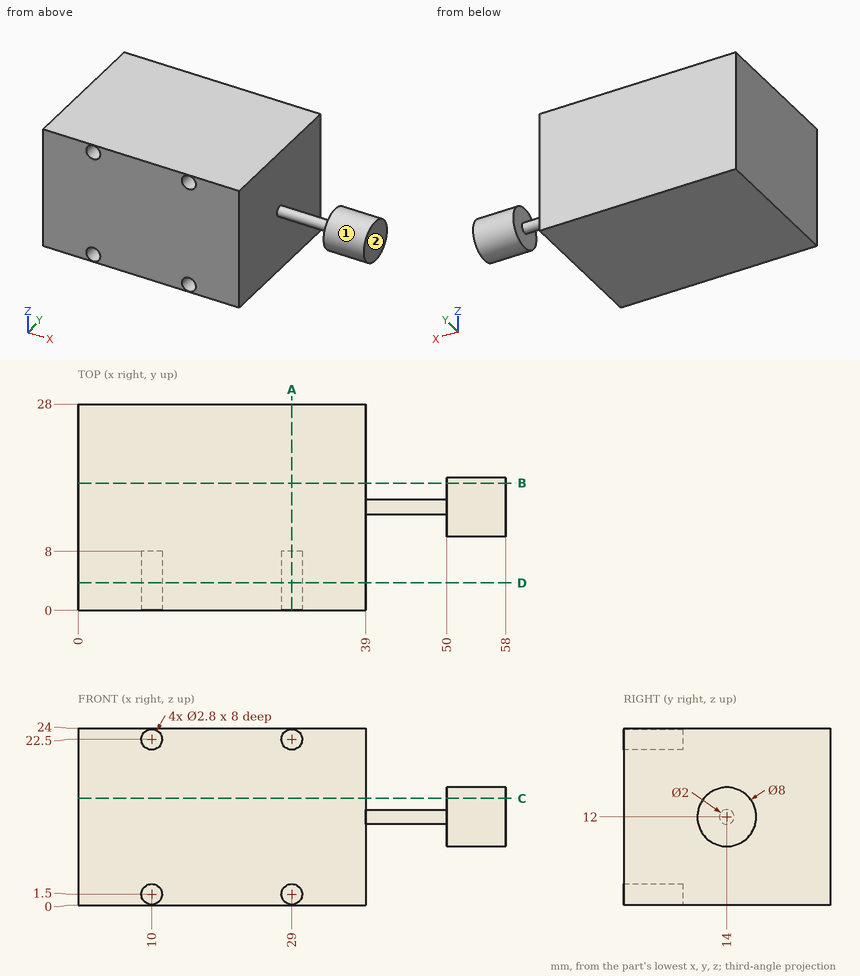
Here's the drawing with two shaded views (mm, measured from the low corner). I have some questions. A direction names the side the tool comes from. Give positions to 0.01 mm unless a question says otherwise; leave off trailing zeros. Loops run counter-clockwise (first coordinate to the right, second up) from the corner with the lowest first, then second, coordinate; pieces in that order, holes last. Notation, with made-up numbers: (-23.5, 8) - (5.5, 8) arc R31 ccw to (5.5, 40) - close; hole circle Ø6 at (38, 88). An arc over 180 degrees is marked (long way). One line per item, written item: value.
(1) I need wall thicknesses on line 1 along X through (y, z) = (2, 1.5); line 2 along Z through (x, y) = (11, 6.25); line 3 along X through (y, z) = (10, 13.75). Which ranges of each line are inside material? Lowest first, please.
Verdict:
line 1: 0 to 8.6, 11.4 to 27.6, 30.4 to 39
line 2: 0 to 0.52, 2.48 to 21.52, 23.48 to 24
line 3: 0 to 39
(2) If we section it at C-C, the plane z = 14.5: List the corners of the cut face in (x, y) for me, plus the area to 3 significant figures.
Verdict:
outline: (0, 0) - (39, 0) - (39, 28) - (0, 28) - close; (50, 10.88) - (58, 10.88) - (58, 17.12) - (50, 17.12) - close
area: 1,140 mm^2
(3) If we section it at D-D, the plane y = 3.75: List the corners of the cut face in (x, z) for me.
Verdict:
outline: (0, 0) - (39, 0) - (39, 24) - (0, 24) - close; hole circle Ø2.8 at (10, 1.5); hole circle Ø2.8 at (10, 22.5); hole circle Ø2.8 at (29, 1.5); hole circle Ø2.8 at (29, 22.5)
(4) If we section it at B-B, the plane y = 17.25: List the corners of the cut face in (x, z) for me.
Verdict:
outline: (0, 0) - (39, 0) - (39, 24) - (0, 24) - close; (50, 9.67) - (58, 9.67) - (58, 14.33) - (50, 14.33) - close
(5) I'm going to push flat-ended pins straight in: pin 1 (1.4 mm diameter, centred on x = 10, z = 22, fed in from -Y); pin 2 (1 mm diameter, centred on y = 22.5, z = 14, fed in from +X). Where does each tip first touch, or does it pass through?
Verdict:
pin 1: y = 8
pin 2: x = 39
(6) On a 3-axis mill with a long thin cutter (end or side, diameter ignored), from which of +Z, -Z, +X, -X, +Y, -Y can I reach the whole of each face in a straight line? I mean the marked faces 1 and 2. Say none if no direction works.
Verdict:
face 1: +X
face 2: +Z, -Z, +X, +Y, -Y
(7) If we section it at A-A, the plane x = 29: List the corners of the cut face in (y, z) for me, plus the area to 3 significant figures.
Verdict:
outline: (0, 0) - (28, 0) - (28, 24) - (0, 24) - (0, 23.9) - (8, 23.9) - (8, 21.1) - (0, 21.1) - (0, 2.9) - (8, 2.9) - (8, 0.1) - (0, 0.1) - close
area: 627 mm^2
